Autodesk Inventor part; units mm, degrees
ref_plane "YZ Plane" through (0, 0, 0) normal (1, 0, 0) x (0, 1, 0)
ref_plane "XZ Plane" through (0, 0, 0) normal (0, 1, 0) x (-1, 0, 0)
ref_plane "XY Plane" through (0, 0, 0) normal (0, 0, 1) x (1, 0, 0)
sketch "Sketch1" plane through (0, 0, 0) normal (0, 0, 1) x (1, 0, 0)
  line L0 (0, 0) -> (120, 0)
  line L1 (120, 0) -> (120, 50)
  line L2 (120, 50) -> (0, 50)
  line L3 (0, 50) -> (0, 0)
  dimension "d0" = 120
  dimension "d1" = 50
extrude "Extrusion1" add sketch "Sketch1" along normal blind 10
sketch "Sketch2" plane through (0, 0, 10) normal (0, 0, 1) x (1, 0, 0)
  line L0 (0, 50) -> (0, 0)
  line L1 (0, 11.5) -> (0, 38.5)
  line L2 (0, 38.5) -> (27.5, 38.5)
  line L3 (30, 36) -> (30, 14)
  line L4 (27.5, 11.5) -> (0, 11.5)
  line L5 (0, 11.5) -> (0, 38.5)
  arc A0 (30, 36) -> (27.5, 38.5) centre (27.5, 36) ccw
  arc A1 (27.5, 11.5) -> (30, 14) centre (27.5, 14) ccw
  point P0 (0, 25)
  point P1 (30, 11.5)
  point P2 (30, 38.5)
  dimension "d4" = 27
  dimension "d5" = 30
  dimension "d8" = 2.5
  dimension "d9" = 2.5
extrude "Extrusion2" cut sketch "Sketch2" against normal blind 1
sketch "Sketch3" plane through (0, 0, 9) normal (0, 0, 1) x (1, 0, 0)
  arc A0 (30, 36) -> (27.5, 38.5) centre (27.5, 36) ccw
  line L0 (0, 38.5) -> (27.5, 38.5)
  line L1 (0, 38.5) -> (27.5, 38.5)
  line L2 (0, 11.5) -> (0, 38.5)
  line L3 (27.5, 11.5) -> (0, 11.5)
  arc A1 (27.5, 11.5) -> (30, 14) centre (27.5, 14) ccw
  line L4 (30, 36) -> (30, 14)
  arc A2 (30, 36) -> (27.5, 38.5) centre (27.5, 36) ccw
  line L5 (30, 36) -> (30, 14)
  line L6 (30, 38.5) -> (22, 38.5)
  line L7 (22, 38.5) -> (22, 33.25)
  line L8 (22, 33.25) -> (30, 33.25)
  line L9 (30, 33.25) -> (30, 38.5)
  circle A3 centre (22, 33.25) radius 1.75
  line L10 (30, 38.5) -> (8, 38.5)
  line L11 (8, 38.5) -> (8, 33.25)
  line L12 (8, 33.25) -> (30, 33.25)
  line L13 (30, 33.25) -> (30, 38.5)
  circle A4 centre (8, 33.25) radius 1.75
  line L14 (30, 25) -> (16.651, 25)
  circle A5 centre (22, 16.75) radius 1.75
  circle A6 centre (8, 16.75) radius 1.75
  point P0 (0, 0)
  dimension "d10" = 8
  dimension "d11" = 5.25
  dimension "d12" = 3.5
  dimension "d13" = 22
  dimension "d14" = 3.5
extrude "Extrusion3" cut sketch "Sketch3" against normal up to surface (9 mm away) contours A3 L12 L8 | L8 L7 A3 | L7 L12 A3 | A4 L12 L11 | L11 L12 A4 | A5 | A6
ref_plane "Work Plane1" through (60, 0, 0) normal (-1, 0, 0) x (0, 0, 1)
mirror "Mirror1" about plane through (60, 0, 0) normal (-1, 0, 0) of "Extrusion2", "Extrusion3"
ref_plane "Work Plane2" through (0, 25, 0) normal (0, -1, 0) x (1, 0, 0)
sketch "Sketch6" plane through (0, 0, 0) normal (-1, 0, 0) x (0, 0, 1)
  line L0 (9, 38.5) -> (10, 38.5)
  line L1 (9, 11.5) -> (9, 38.5)
  line L2 (10, 11.5) -> (9, 11.5)
  line L3 (0, 50) -> (0, 0)
  line L4 (0, 0) -> (10, 0)
  line L5 (10, 11.5) -> (10, 0)
  line L6 (0, 50) -> (10, 50)
  line L7 (10, 50) -> (10, 38.5)
extrude "Extrusion6" add sketch "Sketch6" along normal blind 3
mirror "Mirror4" about plane through (60, 0, 0) normal (-1, 0, 0) of "Extrusion6"
sketch "Sketch7" plane through (0, 0, 0) normal (0, 0, -1) x (-1, 0, 0)
  circle A0 centre (-112, 16.75) radius 1.75
  circle A1 centre (-112, 16.75) radius 3.25
  point P0 (0, 0)
  dimension "d27" = 6.5
extrude "Extrusion7" cut sketch "Sketch7" against normal blind 4
pattern_linear "Rectangular Pattern1" count 2 spacing -14 along (1, 0, 0) count 2 spacing 16.5 along (0, 1, 0) of "Extrusion7"
mirror "Mirror5" about plane through (60, 0, 0) normal (-1, 0, 0) of "Extrusion7", "Rectangular Pattern1"
sketch "Sketch9" plane through (-3, 0, 0) normal (-1, 0, 0) x (0, 0, 1)
  line L0 (10, 50) -> (5, 50)
  line L1 (5, 50) -> (5, 44)
  line L2 (5, 44) -> (10, 44)
  line L3 (10, 44) -> (10, 50)
  circle A0 centre (5, 44) radius 2.05
  point P0 (0, 0)
  dimension "d36" = 5
  dimension "d37" = 6
  dimension "d38" = 4.1
extrude "Extrusion8" cut sketch "Sketch9" against normal blind 5.5 contours A0 L2 L1 | L1 L2 A0
mirror "Mirror6" about plane through (0, 25, 0) normal (0, -1, 0) of "Extrusion8"
sketch "Sketch12" plane through (0, 0, 0) normal (0, 0, -1) x (-1, 0, 0)
  line L0 (-123, 0) -> (3, 0)
  line L1 (-60, 0) -> (-60, 50)
  line L2 (3, 50) -> (-123, 50)
  line L3 (-88, 5) -> (-88, 45)
  line L4 (-88, 45) -> (-32, 45)
  line L5 (-32, 45) -> (-32, 5)
  line L6 (-32, 5) -> (-88, 5)
  line L7 (-88, 5) -> (-32, 45) construction
  line L8 (-88, 45) -> (-32, 5) construction
  line L9 (-60, 45) -> (-60, 43)
  line L10 (-63.9713, 27.8366) -> (-62.8088, 29.4641)
  line L11 (-62.8088, 29.4641) -> (-85.7421, 45.845)
  line L12 (-63.8051, 43) -> (-81.7591, 43)
  line L13 (-60, 43) -> (-60, 27.1502)
  line L14 (-62.8088, 29.4641) -> (-60, 27.1502)
  line L15 (-88, 25) -> (-86, 25)
  line L16 (-86, 25) -> (-86, 27)
  line L17 (-79.67, 39.05) -> (-80.8325, 37.4226)
  line L18 (-80.8325, 37.4226) -> (-69.7179, 29.4835)
  line L19 (-86, 41.1136) -> (-86, 27)
  line L20 (-86, 41.1136) -> (-80.8325, 37.4226)
  line L21 (-69.7179, 29.4835) -> (-63.4409, 25)
  line L22 (-63.4409, 25) -> (-86, 25)
  line L23 (-63.8051, 43) -> (-60, 43)
  line L24 (-57.1912, 29.4641) -> (-34.2579, 45.845)
  line L25 (-56.1949, 43) -> (-38.2409, 43)
  line L26 (-57.1912, 29.4641) -> (-60, 27.1502)
  line L27 (-34, 25) -> (-34, 27)
  line L28 (-39.1675, 37.4226) -> (-50.2821, 29.4835)
  line L29 (-34, 41.1136) -> (-34, 27)
  line L30 (-34, 41.1136) -> (-39.1675, 37.4226)
  line L31 (-50.2821, 29.4835) -> (-56.5591, 25)
  line L32 (-56.5591, 25) -> (-34, 25)
  line L33 (-56.1949, 43) -> (-60, 43)
  line L34 (-88, 5) -> (-32, 45) construction
  line L35 (-62.8088, 20.5359) -> (-85.7421, 4.155)
  line L36 (-63.8051, 7) -> (-81.7591, 7)
  line L37 (-62.8088, 20.5359) -> (-60, 22.8498)
  line L38 (-86, 25) -> (-86, 23)
  line L39 (-80.8325, 12.5774) -> (-69.7179, 20.5165)
  line L40 (-86, 8.8864) -> (-86, 23)
  line L41 (-86, 8.8864) -> (-80.8325, 12.5774)
  line L42 (-69.7179, 20.5165) -> (-63.4409, 25)
  line L43 (-34, 25) -> (-34, 23)
  line L44 (-34, 8.8864) -> (-34, 23)
  line L45 (-34, 8.8864) -> (-39.1675, 12.5774)
  line L46 (-39.1675, 12.5774) -> (-50.2821, 20.5165)
  line L47 (-50.2821, 20.5165) -> (-56.5591, 25)
  line L48 (-57.1912, 20.5359) -> (-34.2579, 4.155)
  line L49 (-56.1949, 7) -> (-38.2409, 7)
  line L50 (-56.1949, 7) -> (-60, 7)
  line L51 (-57.1912, 20.5359) -> (-60, 22.8498)
  line L52 (-60, 7) -> (-63.8051, 7)
  point P0 (0, 0)
  point P1 (-60, 25)
  dimension "d41" = 40
  dimension "d42" = 56
  dimension "d43" = 2
  dimension "d45" = 2
  dimension "d46" = 2
  dimension "d47" = 2
  dimension "d48" = 2
extrude "Extrusion9" cut sketch "Sketch12" against normal up to surface (10 mm away) contours L52 L36 L35 L37 L1 | L1 L51 L48 L49 L50 | L16 L19 L20 L18 L21 L22 | L22 L42 L39 L41 L40 L38 | L14 L11 L12 L23 L1 | L1 L33 L25 L24 L26 | L32 L31 L28 L30 L29 L27 | L43 L44 L45 L46 L47 L32
sketch "Sketch13" plane through (-3, 50, 10) normal (0, 1, 0) x (1, 0, 0)
  line L0 (126, 0) -> (126, 10)
  line L1 (0, 10) -> (126, 10)
  line L2 (0, 0) -> (126, 0)
  line L3 (0, 0) -> (0, 10)
  point P0 (3, 10)
extrude "Extrusion10" add sketch "Sketch13" along normal blind 5
mirror "Mirror7" about plane through (0, 25, 0) normal (0, -1, 0) of "Extrusion10"
mirror "Mirror8" about plane through (60, 0, 0) normal (-1, 0, 0) of "Extrusion8", "Mirror6"
sketch "Sketch14" plane through (-3, 55, 10) normal (0, 1, 0) x (1, 0, 0)
  line L0 (0, 0) -> (126, 0)
  line L1 (0, 0) -> (126, 0)
  line L2 (126, 0) -> (126, 10)
  line L3 (126, 10) -> (0, 10)
  line L4 (0, 10) -> (0, 0)
  point P0 (3, 10)
extrude "Extrusion11" add sketch "Sketch14" along normal blind 1
mirror "Mirror9" about plane through (0, 25, 0) normal (0, -1, 0) of "Extrusion11"
Geometry check sheet. Reference: the model listing, model coordinates, mm. A direction names the side the tool comes from. Round coordinates to 2 decimals unless told otherwise and drop trailing zeros. Order: outer loops, then holes, each group sorted by start corner. A loop starts at its lowest first (then second) coordinate and runs counter-clockwise, first axis right, second up. Notation, with made-up numbers: M -37,74 L 0,74 A33 cw 0,102 Z; hole C 69.5,72 d7. An arc over 180 degrees is marked long. Answer in a Markdown table with one row per item. Add a question column.
Item 1: Depth check by flat-ended pin: pin 1 Ø6 at (x, y) = (8, 16.75) entering from +Z; pin 2 Ø4 at (x, y) = (112, 16.75) entering from -Z; pin 3 Ø2 at (y, z) = (44, 4) entering from +X. Enter the tip coordinate at first touch or a pass-through.
Item 2: Sectioned sample at B-B, the plane x = 17. Enter the section's corners in (y, z), plus the area to 3 significant figures.
Item 3: Set-up check for faces 4 (the face through (7.295, 36.423, 1.972)), 5 (the face through (58.58, 28.32, 4.93)), 6 (the face through (14, 25, 9)), 7 (the face through (90.713, 12.252, 9.507)): record each of +Z, -Z, +X, -X, +Y, -Y from which the full face is reachable in a straight line by a thin tool's end or side.
Item 4: Sectioned sample at C-C, the plane x = 68.5. Enter the section's corners in (y, z).
Item 5: Sectioned sample at A-A, the plane x = 98. Enter the section's corners in (y, z), plus the area to 3 significant figures.
Item 6: Sectioned sample at D-D, the plane y = 33.25. State how many separate pieces and enclosed holes the cut face has, plus the area to 3 significant figures.
Item 7: Material ranges on L1, parallel to Y at x = -0.7, z = 5; L2, parallel to Y at x = 58.5, z = 9; L3, parallel to X at y = 12.5, z = 4, recorded low to high. Write a range as [from, to].
Item 8: Draft check along Z on faces 1 (the face through (20.25, 33.33, 6.54)), 2 (the face through (106, 25, 9)), 3 (the face through (120.288, 41.967, 4.733)). Enter one of: released by +Z, released by -Z, zero draft, split by the parting line, or undercut.
Filled in:
| question | item | result |
|---|---|---|
| 1 | pin 1 | stops at z = 9 |
| 1 | pin 2 | stops at z = 4 |
| 1 | pin 3 | stops at x = 117.5 |
| 2 | outline | M -6,0 L 56,0 L 56,10 L 38.5,10 L 38.5,9 L 11.5,9 L 11.5,10 L -6,10 Z |
| 2 | area | 593 mm² |
| 3 | face 4 | -Z |
| 3 | face 5 | +Z, -Z |
| 3 | face 6 | +Z, -X |
| 3 | face 7 | +Z, +X |
| 4 | outline | M -6,0 L 7,0 L 7,10 L -6,10 Z; M 16.47,0 L 21.39,0 L 21.39,10 L 16.47,10 Z; M 28.61,0 L 33.53,0 L 33.53,10 L 28.61,10 Z; M 43,0 L 56,0 L 56,10 L 43,10 Z |
| 5 | outline | M -6,0 L 13.5,0 L 13.5,4 L 15,4 L 15,9 L 11.5,9 L 11.5,10 L -6,10 Z; M 18.5,4 L 20,4 L 20,0 L 30,0 L 30,4 L 31.5,4 L 31.5,9 L 18.5,9 Z; M 35,4 L 36.5,4 L 36.5,0 L 56,0 L 56,10 L 38.5,10 L 38.5,9 L 35,9 Z |
| 5 | area | 506 mm² |
| 6 | separate pieces | 8 |
| 6 | enclosed holes | 0 |
| 6 | area | 638 mm² |
| 7 | L1 | y = [-6, 3.95], [8.05, 41.95], [46.05, 56] |
| 7 | L2 | y = [-6, 7], [21.61, 28.39], [43, 56] |
| 7 | L3 | x = [-3, 34], [39.06, 45.94], [74.06, 80.94], [86, 123] |
| 8 | face 1 | zero draft |
| 8 | face 2 | released by +Z |
| 8 | face 3 | undercut |
